Autodesk Fusion 360 part; units mm, degrees
sketch "Sketch1" plane through (0, 0, 0) normal (0, 0, 1) x (1, 0, 0)
  line L0 (0, 0) -> (26, 0)
  line L1 (26, 0) -> (26, 6.2)
  line L2 (26, 6.2) -> (0, 6.2)
  line L3 (0, 6.2) -> (0, 0)
  dimension "d1" = 26
  dimension "d2" = 6.2
extrude "Extrude1" add sketch "Sketch1" along normal blind 3
sketch "Sketch2" plane through (0, 0, 0) normal (0, 0, 1) x (1, 0, 0)
  line L0 (0, 0) -> (13, 0)
  line L1 (13, 0) -> (13, -3.2)
  line L2 (13, -3.2) -> (9.8, -3.2)
  line L3 (9.8, -3.2) -> (9.8, 0)
  line L4 (9.8, 0) -> (13, 0)
  line L5 (13, 0) -> (13, -3.2)
  line L6 (13, -3.2) -> (16.2, -3.2)
  line L7 (16.2, -3.2) -> (16.2, 0)
  line L8 (16.2, 0) -> (13, 0)
  line L9 (13, 0) -> (13, -3.2)
  line L10 (9.8, -3.2) -> (16.2, -3.2)
  line L11 (16.2, -3.2) -> (16.2, 18.8)
  line L12 (16.2, 18.8) -> (9.8, 18.8)
  line L13 (9.8, 18.8) -> (9.8, -3.2)
  dimension "d5" = 13
  dimension "d6" = 3.2
  dimension "d7" = 3.2
  dimension "d8" = 3.2
  dimension "d9" = 6.4
  dimension "d10" = 22
extrude "Extrude2" add sketch "Sketch2" along normal blind 13.4
sketch "Sketch3" plane through (0, -3.2, 0) normal (0, -1, 0) x (1, 0, 0)
  line L0 (9.8, 0) -> (16.2, 0)
  line L1 (16.2, 0) -> (16.2, 13.4)
  line L2 (16.2, 13.4) -> (9.8, 13.4)
  line L3 (9.8, 13.4) -> (9.8, 0)
  line L4 (9.8, 13.4) -> (13, 13.4)
  line L5 (13, 13.4) -> (13, 0)
  line L6 (13, 0) -> (9.8, 0)
  line L7 (9.8, 0) -> (9.8, 13.4)
extrude "Extrude3" add sketch "Sketch3" along normal blind 6.2 contours L0 L2 L3 L4 L5 L6 L7
sketch "Sketch4" plane through (0, 0, 3) normal (0, 0, 1) x (-1, 0, 0)
  line L0 (-9.8, 0) -> (-9.8, -6.2)
  line L1 (-9.8, -6.2) -> (0, -6.2)
  line L2 (0, -6.2) -> (0, 0)
  line L3 (0, 0) -> (-9.8, 0)
  line L4 (-13, 3) -> (-13, -19)
  line L5 (-13, -19) -> (-13, 3)
  line L6 (0, -3.1) -> (-26, -3.1)
  line L7 (-13, -3.1) -> (-3.5, -3.1)
  line L8 (-13, -3.1) -> (-22.5, -3.1)
  circle A0 centre (-3.5, -3.1) radius 1.6
  circle A1 centre (-22.5, -3.1) radius 1.6
  dimension "d15" = 9.5
  dimension "d16" = 9.5
  dimension "d17" = 3.2
  dimension "d18" = 3.2
extrude "Extrude4" cut sketch "Sketch4" against normal blind 17 contours L6 L8 A1 | L6 L8 A1 | L6 L7 A0 | L6 L7 A0
sketch "Sketch5" plane through (9.8, 0, 0) normal (-1, 0, 0) x (0, -1, 0)
  line L0 (-6.2, 0) -> (-6.2, 3)
  line L1 (-6.2, 3) -> (0, 3)
  line L2 (0, 3) -> (0, 0)
  line L3 (0, 0) -> (9.4, 0)
  line L4 (9.4, 0) -> (9.4, 13.4)
  line L5 (9.4, 13.4) -> (-18.8, 13.4)
  line L6 (-18.8, 13.4) -> (-18.8, 0)
  line L7 (-18.8, 0) -> (-6.2, 0)
  line L8 (-18.8, 6.7) -> (-9.8, 6.7)
  line L9 (-9.8, 6.7) -> (-9.8, 9.2)
  line L10 (-9.8, 9.2) -> (-18.8, 9.2)
  line L11 (-18.8, 9.2) -> (-18.8, 6.7)
  line L12 (-18.8, 6.7) -> (-9.8, 6.7)
  line L13 (-9.8, 6.7) -> (-9.8, 4.2)
  line L14 (-9.8, 4.2) -> (-18.8, 4.2)
  line L15 (-18.8, 4.2) -> (-18.8, 6.7)
  dimension "d21" = 9
  dimension "d22" = 2.5
  dimension "d23" = 2.5
extrude "Extrude5" cut sketch "Sketch5" against normal blind 17 contours L6 L8 L12 L13 L14 L15 | L6 L8 L9 L10 L11 L12
sketch "Sketch6" plane through (0, 0, 4.2) normal (0, 0, 1) x (-1, 0, 0)
  line L0 (-16.2, -9.8) -> (-16.2, -18.8)
  line L1 (-16.2, -18.8) -> (-9.8, -18.8)
  line L2 (-9.8, -18.8) -> (-9.8, -9.8)
  line L3 (-9.8, -9.8) -> (-16.2, -9.8)
  line L4 (-13, -3) -> (-13, -16)
  circle A0 centre (-13, -16) radius 2.5
  dimension "d26" = 13
  dimension "d27" = 5
extrude "Extrude6" cut sketch "Sketch6" against normal blind 1 contours A0
Input: part model. Units: mm. Frame: model coordinates. A direction names the side the tool comes from. Round coordinates to 2 decimals unless told otherwise and drop trailing zeros. Write each loop counter-clockwise with the first axis right and the second up, starting at its lowest first coordinate (ties: lowest second). Pieces come first, ordered by that corner, then holes. Notation, with made-up numbers: M -37.75,-14 L -21.75,-14 A10 cw -21.75,-10 Z; hole C -32.5,21 d4. An arc over 180 degrees is marked long. Write each question's results on one line, items separated by ' | '.
Q1. Draft query along X for faces 5 (the face through (13, 16, 3.2)), 6 (the face through (11, -9.4, 7)), 7 (the face through (0, 3, 1)). Return one class per face: released by +X, released by -X, zero draft, split by the parting line, or undercut.
Results:
face 5: undercut | face 6: zero draft | face 7: released by -X
Q2. Section query B-B (y = 3.1). Return loops of the section in (x, z).
Results:
outline: M 0,0 L 1.9,0 L 1.9,3 L 0,3 Z; M 5.1,0 L 20.9,0 L 20.9,3 L 16.2,3 L 16.2,13.4 L 9.8,13.4 L 9.8,3 L 5.1,3 Z; M 24.1,0 L 26,0 L 26,3 L 24.1,3 Z
Q3. Pin query (flat end, axial travel): P1, Ø4, axis at y = -2, z = 9.5, coming from the -X side; P2, Ø1.9, axis at x = 20, y = 2.5, coming from the +Z side; P3, Ø2.5, axis at x = 4, z = 1, coming from the +Y side; P4, Ø3, axis at x = 13, y = 14, coming from the -Z side. Return the tip coordinate at first contact, or that it passes through.
Results:
P1: stops at x = 9.8 | P2: stops at z = 3 | P3: stops at y = 6.2 | P4: stops at z = 0
Q4. Line query: line 1 along X through (y, z) = (3.1, 0.9); line 2 along Y through (x, z) = (22.5, 1.7); line 3 along Z through (x, y) = (14.25, 12). Output: solid intervals per line, ascending.
Results:
line 1: x = 0 to 1.9, 5.1 to 20.9, 24.1 to 26 | line 2: y = 0 to 1.5, 4.7 to 6.2 | line 3: z = 0 to 4.2, 9.2 to 13.4
Q5. Section query A-A (y = 16). Return loops of the section in (x, z), and give its area (3 significant figures).
Results:
outline: M 9.8,0 L 16.2,0 L 16.2,4.2 L 15.5,4.2 L 15.5,3.2 L 10.5,3.2 L 10.5,4.2 L 9.8,4.2 Z; M 9.8,9.2 L 16.2,9.2 L 16.2,13.4 L 9.8,13.4 Z | area: 48.8 mm^2
Q6. Access query for faces 1 (the face through (13, 14, 9.2)), 2 (the face through (6, 3, 3)), 3 (the face through (5, 0, 1)), 4 (the face through (21, 0, 1)). Directions: +Z, -Z, +X, -X, +Y, -Y. A direction counts if a zero-diameter tool reaches every point of the face in a straight line with its end or side. Return the directions, or none.
Results:
face 1: +X, -X, +Y | face 2: +Z, -X, +Y, -Y | face 3: +Z, -Z, -X, -Y | face 4: +Z, -Z, +X, -Y
Q7. Section query C-C (x = 22.5). Return loops of the section in (y, z).
Results:
outline: M 0,0 L 1.5,0 L 1.5,3 L 0,3 Z; M 4.7,0 L 6.2,0 L 6.2,3 L 4.7,3 Z
Q8. Section query D-D (z = 5.25). Return loops of the section in (x, y).
Results:
outline: M 9.8,-9.4 L 13,-9.4 L 13,-3.2 L 16.2,-3.2 L 16.2,9.8 L 9.8,9.8 Z
